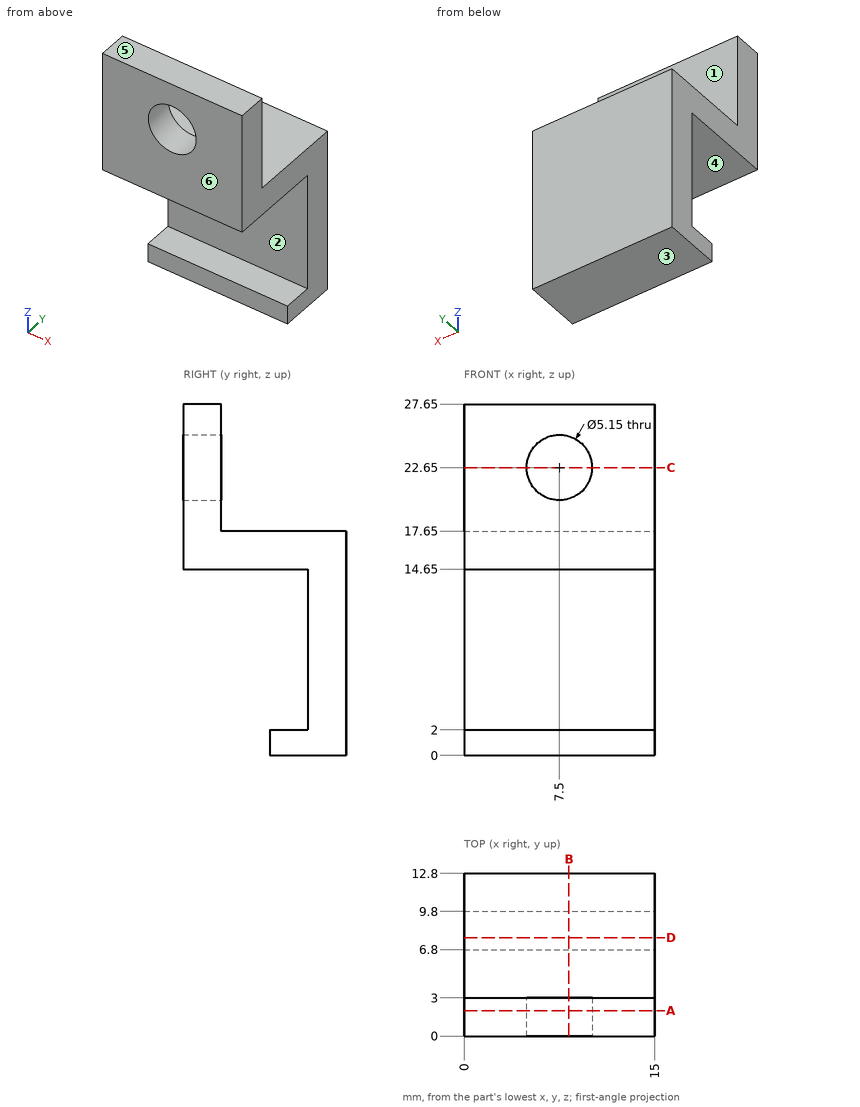
Input: dimensioned drawing with shaded views. Units: mm. Origin: part minimum x, y, z. A direction names the side the tool comes from. Coordinates: 2 decimals unless noted, no trailing zeros. Order: outer loops, then holes, each group sorted by start corner. A loop starts at its lowest first (then second) coordinate and runs counter-clockwise, first axis right, second up.
Item 1: Material intervals for line 1 along Z through (x, y) = (10.75, 9); line 2 along X through (y, z) = (1.6, 22.65) (3 decimals); line 3 along Z through (x, y) = (7.5, 1.2) (3 decimals), sorted ascending.
Answer:
line 1: z = 0 to 2, 14.65 to 17.65
line 2: x = 0 to 4.925, 10.075 to 15
line 3: z = 14.65 to 20.075, 25.225 to 27.65
Item 2: Section query C-C (z = 22.65). Output: boundary loops of the cut face in (x, y) (3 decimals), then the cut area to 4 significant figures.
Answer:
outline: (0, 0) - (4.925, 0) - (4.925, 3) - (0, 3) - close; (10.075, 0) - (15, 0) - (15, 3) - (10.075, 3) - close
area: 29.55 mm2
Item 3: Section query A-A (y = 2). Output: boundary loops of the cut face in (x, z) (3 decimals).
Answer:
outline: (0, 14.65) - (15, 14.65) - (15, 27.65) - (0, 27.65) - close; hole circle Ø5.15 at (7.5, 22.65)
Item 4: Section query B-B (x = 8.25). Output: boundary loops of the cut face in (y, z).
Answer:
outline: (0, 14.65) - (9.8, 14.65) - (9.8, 2) - (6.8, 2) - (6.8, 0) - (12.8, 0) - (12.8, 17.65) - (3, 17.65) - (3, 20.19) - (0, 20.19) - close; (0, 25.11) - (3, 25.11) - (3, 27.65) - (0, 27.65) - close
Item 5: Section query D-D (y = 7.75). Output: boundary loops of the cut face in (x, z).
Answer:
outline: (0, 0) - (15, 0) - (15, 2) - (0, 2) - close; (0, 14.65) - (15, 14.65) - (15, 17.65) - (0, 17.65) - close
Item 6: Draft query along Z for the marked faces 4, 5 and 6. Return one class per face: released by +Z, released by -Z, zero draft, split by the parting line, or undercut.
Answer:
face 4: undercut
face 5: released by +Z
face 6: zero draft
Item 7: Access query for the marked faces 1, 2 and 3. Directions: +Z, -Z, +X, -X, +Y, -Y. A direction counts if a zero-diameter tool reaches every point of the face in a straight line with its end or side. Return the directions, or none.
Answer:
face 1: +Z, +X, -X, +Y
face 2: +X, -X, -Y
face 3: -Z, +X, -X, +Y, -Y
Item 8: Contact query for flat-ended pins moving along their axis: P1, Ø6, axis at x = 3.5, z = 6.5, coming from the -Y side; P2, Ø1.5, axis at x = 5.5, y = 8, coming from the +Z side; P3, Ø8, axis at x = 5.5, z = 24.5, coming from the +Y side. Output: stop coordinate, or through.
Answer:
P1: stops at y = 9.8
P2: stops at z = 17.65
P3: stops at y = 3
